```python
from build123d import *

# Parameters (mm, degrees)
SKETCH1_W           = 66.04
SKETCH1_H           = 5.08
BOSS_EXTRUDE1_DEPTH = 3.81
SKETCH2_W           = 4.572
SKETCH2_H           = 3.048
CUT_EXTRUDE1_DEPTH  = 6.08
CHAMFER1_SIZE       = 0.254
CUT_EXTRUDE2_DEPTH  = 6.08
SKETCH5_W           = 12.916630293
SKETCH5_H           = 3.048
CUT_EXTRUDE3_DEPTH  = 6.08
SKETCH6_W           = 3.81
SKETCH6_H           = 1.726747829
CUT_EXTRUDE4_DEPTH  = 6.08


with BuildPart() as part:
    # Sketch1 → Boss-Extrude1 (new body)
    with BuildSketch(Plane(origin=(0, 0, 0), x_dir=(1, 0, 0), z_dir=(0, 1, 0))):
        with Locations((-87.329253942, 35.396987703)):
            Rectangle(SKETCH1_W, SKETCH1_H)
    extrude(amount=BOSS_EXTRUDE1_DEPTH)

    # Sketch2 → Cut-Extrude1 (cut, through all)
    with BuildSketch(Plane.XY.offset(-32.856987703)):
        with Locations((-60.405253942, 2.286)):
            Rectangle(SKETCH2_W, SKETCH2_H)
    extrude(amount=-CUT_EXTRUDE1_DEPTH, mode=Mode.SUBTRACT)

    # Chamfer1
    chamfer1_edges = [part.edges().sort_by_distance(p)[0] for p in [
        (-54.309253942, 3.81, -35.396987703),
        (-58.119253942, 3.81, -35.396987703),
    ]]
    chamfer(chamfer1_edges, length=CHAMFER1_SIZE)

    # Sketch4 → Cut-Extrude2 (cut, through all)
    with BuildSketch(Plane.XY.offset(-32.856987703)):
        Polygon((-64.575422666, 0.762), (-65.794622666, 0.762), (-66.403478406, 1.95694667), (-66.477713127, 2.338851205), (-66.969636987, 2.338851205), (-67.027795569, 2.03965124), (-67.678791391, 0.762), (-68.855851308, 0.762), (-69.464707047, 1.95694667), (-69.522865629, 2.256146635), (-70.030865629, 2.256146635), (-70.089024211, 1.95694667), (-70.69787995, 0.762), (-71.91707995, 0.762), (-72.525935689, 1.95694667), (-72.584094271, 2.256146635), (-73.092094271, 2.256146635), (-73.150252852, 1.95694667), (-73.759108591, 0.762), (-74.978308591, 0.762), (-75.58716433, 1.95694667), (-75.645322912, 2.256146635), (-76.153322912, 2.256146635), (-76.211481494, 1.95694667), (-76.820337233, 0.762), (-78.039537233, 0.762), (-78.648392972, 1.95694667), (-78.706551554, 2.256146635), (-79.214551554, 2.256146635), (-79.272710136, 1.95694667), (-79.881565875, 0.762), (-81.100765875, 0.762), (-81.709621614, 1.95694667), (-81.767780195, 2.256146635), (-82.275780195, 2.256146635), (-82.333938777, 1.95694667), (-82.942794516, 0.762), (-84.161994516, 0.762), (-84.770850255, 1.95694667), (-84.829008837, 2.256146635), (-85.337008837, 2.256146635), (-85.395167419, 1.95694667), (-86.004023158, 0.762), (-87.223223158, 0.762), (-87.832078897, 1.95694667), (-87.890237479, 2.256146635), (-88.398237479, 2.256146635), (-88.45639606, 1.95694667), (-89.065251799, 0.762), (-90.284451799, 0.762), (-90.893307538, 1.95694667), (-90.95146612, 2.256146635), (-91.45946612, 2.256146635), (-91.517624702, 1.95694667), (-92.126480441, 0.762), (-93.345680441, 0.762), (-93.95453618, 1.95694667), (-94.012694762, 2.256146635), (-94.520694762, 2.256146635), (-94.578853344, 1.95694667), (-95.187709083, 0.762), (-96.406909083, 0.762), (-97.015764822, 1.95694667), (-97.073923403, 2.256146635), (-97.581923403, 2.256146635), (-97.640081985, 1.95694667), (-98.248937724, 0.762), (-99.468137724, 0.762), (-100.076993463, 1.95694667), (-100.135152045, 2.256146635), (-100.643152045, 2.256146635), (-100.701310627, 1.95694667), (-101.310166366, 0.762), (-102.529366366, 0.762), (-103.138222105, 1.95694667), (-103.196380687, 2.256146635), (-103.704380687, 2.256146635), (-103.762539268, 1.95694667), (-104.371395007, 0.762), (-105.590595007, 0.762), (-106.199450746, 1.95694667), (-106.257609328, 2.256146635), (-106.765609328, 2.256146635), (-106.82376791, 1.95694667), (-107.432623649, 0.762), (-107.432623649, 3.81), (-106.257609328, 3.81), (-62.691253942, 3.81), (-62.691253942, 0.762), (-63.342249764, 2.03965124), (-63.400408346, 2.338851205), (-63.892332206, 2.338851205), (-63.966566927, 1.95694667), align=None)
    extrude(amount=-CUT_EXTRUDE2_DEPTH, mode=Mode.SUBTRACT)

    # Sketch5 → Cut-Extrude3 (cut, through all)
    with BuildSketch(Plane.XY.offset(-32.856987703)):
        with Locations((-113.890938796, 2.286)):
            Rectangle(SKETCH5_W, SKETCH5_H)
    extrude(amount=-CUT_EXTRUDE3_DEPTH, mode=Mode.SUBTRACT)

    # Sketch6 → Cut-Extrude4 (cut, through all)
    with BuildSketch(Plane.XY.offset(-32.856987703)):
        with Locations((-56.214253942, 3.202225119)):
            Rectangle(SKETCH6_W, SKETCH6_H)
    extrude(amount=-CUT_EXTRUDE4_DEPTH, mode=Mode.SUBTRACT)


solid = part.part
```
The model under review builds one solid part; all positions refer to its coordinate system, in mm. A direction names the side the tool comes from. Round coordinates to 2 decimals unless told otherwise and drop trailing zeros. Write each loop counter-clockwise with the first axis right and the second up, starting at its lowest first coordinate (ties: lowest second). Pieces come first, ordered by that corner, then holes. Notation, with made-up numbers: (86.25, 16) - (96.25, 16) arc R9 cw to (96.25, 29) - close; hole circle Ø10 at (-34, 39.25). An arc over 180 degrees is marked (long way). Answer as CSV lines item,"result". Start each with the question number.
(1) We need section B-B on y = 1.6. Give the number of separate pieces and of enclosed holes in the cut face, plus the area to 3 significant figures.
(2) To check wall thickness, follow line 1 (Y direction, x = -77.5, z = -37.3); line 2 (Y direction, x = -70, z = -34.75). State the ranges of each line that lie inside material, in increasing order.
(3) For pin 1 Ø1 at (x, z) = (-77, -35.5) entering from +Y; pin 2 Ø1 at (x, z) = (-71.5, -35) entering from +Y; pin 3 Ø3 at (x, z) = (-98.5, -35.5) entering from -Y; pin 4 Ø0.6 at (x, z) = (-71.5, -36.5) entering from +Y, all flat-tipped, find the tip position at first contact; note any pin that passes through.
(4) Draft analysis for pull direction X (two halves, no side actions). For faces 1 (the flat face through (-88, 1, -32.857)), 2 (the flat face through (-74, 0.762, -35)), 3 (the flat face through (-107.124, 1.368, -35.361)), 4 (the flat face through (-68, 0.762, -35)), state which applies: pulls with the +X half, pulls with the -X half, needs draft (parallel to the pull), parting line crosses it, or undercut.
(5) We need section A-A on x = -108. State the section outline as (y, z) points, plus the area to 3 significant figures.
(6) For faces 5 (the flat face through (-96.707, 1.351, -35.361)), 6 (the flat face through (-56, 2.339, -35)), list the 3-axis set-ups (+Z, -Z, +X, -X, +Y, -Y) from which the entire face can be reached by the end or side of a thin tool; tool diameter is ignored.
Worked answers:
1,separate pieces,"16"
1,enclosed holes,"0"
1,area,"95.1 mm²"
2,line 1,"0 to 0.76"
2,line 2,"0 to 2.26"
3,pin 1,"y = 1.39"
3,pin 2,"y = 0.92"
3,pin 3,"y = 0"
3,pin 4,"y = 0.76"
4,face 1,"needs draft"
4,face 2,"undercut"
4,face 3,"pulls with the -X half"
4,face 4,"undercut"
5,outline,"(0, -37.94) - (0.76, -37.94) - (0.76, -32.86) - (0, -32.86) - close"
5,area,"3.87 mm²"
6,face 5,"+Z, -Z, +Y"
6,face 6,"+Z, -Z, +X, -X, +Y"
